from build123d import *

# Parameters (mm, degrees)
F0_W     = 18.2879995555
F0_H     = 19.3040007725
F3_D     = 30.48
F3_DEPTH = 16.51
F3_TIP   = 9.157115834
F5_D     = 10.16
F7_D     = 4.6736
F9_D     = 4.6736


with BuildPart() as f1:
    # F0 (on Front) → F1 (revolve)
    with BuildSketch(Plane.XZ):
        with Locations((-9.1439997777, -4.5719998889)):
            Rectangle(F0_W, F0_H)
    revolve(axis=Axis((0, 0, -4.5719998889), (0, 0, -1)))

    # F3 (one way)
    with BuildSketch(Plane.XY):
        with Locations((0, 0)):
            Circle(F3_D / 2)
    extrude(amount=-F3_DEPTH, mode=Mode.SUBTRACT)
    with Locations(Plane.XY):
        with Locations((0, 0)):
            with Locations((0, 0, -(F3_DEPTH + F3_TIP / 2))):  # 118° drill point
                Cone(0, F3_D / 2, F3_TIP, mode=Mode.SUBTRACT)

    # F5 (through all)
    with Locations(Plane(origin=(0, 0, 0), x_dir=(1, 0, 0), z_dir=(0, 0, -1))):
        with Locations((0, 0)):
            Hole(F5_D / 2)

    # F7 (through all)
    with Locations(Plane(origin=(0, 0, 0), x_dir=(1, 0, 0), z_dir=(0, 0, -1))):
        with Locations((-10.9219979495, 0)):
            Hole(F7_D / 2)

    # F9 (through all)
    with Locations(Plane(origin=(0, 0, 0), x_dir=(1, 0, 0), z_dir=(0, 0, -1))):
        with Locations((10.1600009948, 0)):
            Hole(F9_D / 2)


solid = f1.part
Model file for the job. Use its own axes, mm. A direction names the side the tool comes from. Give positions to 0.01 mm unless a question says otherwise; leave off trailing zeros. Loops run counter-clockwise (first coordinate to the right, second up) from the corner with the lowest first, then second, coordinate; pieces in that order, holes last.
1) Pull direction X, two halves, no side cores. Call faces 3 (the cylindrical face through (0.661, -5.037, 2.576)), 4 (the flat face through (-4, -4, 5.08)), 5 (the cylindrical face through (14.51, -11.13, -4.44)), 6 (the cylindrical face through (-3.3, -14.88, -7.01)): +X half, -X half, draft (parallel to the pull), parting line (faces both ways), or undercut.
2) Saw through at D-D (z = 1.75). Write the cut outline in (x, y).
3) Saw through at B-B (y = 0). Write the cut outline in (x, z).
4) Saw through at C-C (y = 4). Write the cut outline in (x, z).
5) Wall check: line 1 (Y direction, x = 12.5, z = -8.5); line 2 (Z direction, x = -14, y = 3); line 3 (X direction, y = 14, z = -4.5). Give the ranges that are in metal, low to high.
6) Tool access for faces 1 (the flat face through (-4, 4, 0)), 2 (the flat face through (7, 14, -14.224)): list every direction of +Z, -Z, +X, -X, +Y, -Y with a clear straight run to the whole face (end or side of a thin tool).
7) Flat gauge pins, fed straight in: pin 1 Ø10 at (y, z) = (10, -8.5) entering from -X; pin 2 Ø12 at (x, y) = (14.5, -4.5) entering from -Z; pin 3 Ø5.5 at (x, y) = (-10.92, 0) entering from -Z; pin 4 Ø1 at (y, z) = (-7, -1.5) entering from -X. Where does each tip first touch, or does it go through?
8) Saw through at A-A (x = 0). Write the cut outline in (y, z), plus the area to 3 significant figures.
Answer block:
1. face 3: undercut
1. face 4: draft
1. face 5: parting line
1. face 6: undercut
2. outline: circle Ø36.58 at (0, 0); hole circle Ø4.67 at (-10.92, 0); hole circle Ø10.16 at (0, 0); hole circle Ø4.67 at (10.16, 0)
3. outline: (-18.29, -14.22) - (-15.24, -14.22) - (-15.24, 0) - (-13.26, 0) - (-13.26, 5.08) - (-18.29, 5.08) - close; (-8.59, 0) - (-5.08, 0) - (-5.08, 5.08) - (-8.59, 5.08) - close; (5.08, 0) - (7.82, 0) - (7.82, 5.08) - (5.08, 5.08) - close; (12.5, 0) - (15.24, 0) - (15.24, -14.22) - (18.29, -14.22) - (18.29, 5.08) - (12.5, 5.08) - close
4. outline: (-17.85, -14.22) - (-14.71, -14.22) - (-14.71, 0) - (-3.13, 0) - (-3.13, 5.08) - (-17.85, 5.08) - close; (3.13, 0) - (14.71, 0) - (14.71, -14.22) - (17.85, -14.22) - (17.85, 5.08) - (3.13, 5.08) - close
5. line 1: y = -13.35 to -8.72, 8.72 to 13.35
5. line 2: z = 0 to 5.08
5. line 3: x = -11.77 to -6.02, 6.02 to 11.77
6. face 1: -Z
6. face 2: -Z, +X, -X, +Y, -Y
7. pin 1: stops at x = -17.59
7. pin 2: stops at z = -14.22
7. pin 3: stops at z = 0
7. pin 4: stops at x = -17.09
8. outline: (-18.29, -14.22) - (-15.24, -14.22) - (-15.24, 0) - (-5.08, 0) - (-5.08, 5.08) - (-18.29, 5.08) - close; (5.08, 0) - (15.24, 0) - (15.24, -14.22) - (18.29, -14.22) - (18.29, 5.08) - (5.08, 5.08) - close
8. area: 221 mm2
